```python
from build123d import *

# Parameters (mm, degrees)
SKETCH_1_R          = 3.073322802
EXTRUDE_1_DEPTH     = 10
SKETCH_2_R          = 3
EXTRUDE_2_DEPTH     = 5
CUT_EXTRUDE_1_DEPTH = 10


with BuildPart() as part:
    # 草图1 → 凸台-拉伸1 (new body)
    with BuildSketch(Plane(origin=(0, 0, 0), x_dir=(1, 0, 0), z_dir=(0, 1, 0))):
        with BuildLine():
            Line((0, 0), (30.73322802, 0))
            Line((30.73322802, 0), (18.141743603, 40.76055825))
            ThreePointArc((18.141743603, 40.76055825), (15.36661401, 42.513286949), (12.591484417, 40.76055825))
            Line((12.591484417, 40.76055825), (0, 0))
        make_face()
        with Locations(Location((15.36661401, 30, 0), (0, 0, 270))):
            Circle(SKETCH_1_R, mode=Mode.SUBTRACT)
    extrude(amount=EXTRUDE_1_DEPTH)

    # 草图2 → 凸台-拉伸2 (add)
    with BuildSketch(Plane.XZ):
        with Locations(Location((15.36661401, -39.439964147, 0), (0, 0, 90))):
            Circle(SKETCH_2_R)
    extrude(amount=EXTRUDE_2_DEPTH)

    # 草图3 → 切除-拉伸1 (cut)
    with BuildSketch(Plane(origin=(0, 10, 0), x_dir=(1, 0, 0), z_dir=(0, 1, 0))):
        with BuildLine():
            Line((13.327100422, 20.21204175), (13.327100422, 24.21204175))
            Line((13.327100422, 24.21204175), (17.327100422, 24.21204175))
            Line((17.327100422, 24.21204175), (17.327100422, 20.21204175))
            ThreePointArc((17.327100422, 20.21204175), (15.327100422, 0.414082779), (13.327100422, 20.21204175))
        make_face()
    extrude(amount=-CUT_EXTRUDE_1_DEPTH, mode=Mode.SUBTRACT)


solid = part.part
```
For this review, take the finished solid that the model builds, in its own axes (mm). A direction names the side the tool comes from. Coordinates: 2 decimals unless noted, no trailing zeros. Write each loop counter-clockwise with the first axis right and the second up, starting at its lowest first coordinate (ties: lowest second). Pieces come first, ordered by that corner, then holes. Notation, with made-up numbers: (89.25, 76) - (100.25, 76) arc R4 cw to (100.25, 82) - close; hole circle Ø10 at (35, 2). An arc over 180 degrees is marked (long way). Answer in a Markdown table with one row per item. Add a question column.
Q1. For probe 1 along Z at (x, y) = (16, 7.75); probe 2 along X at (y, z) = (0.75, -6); probe 3 along X at (y, z) = (2.5, -5.5), list the stretches that pass through material, from the lowest coordinate up.
Q2. For P1, Ø6, axis at y = 2.5, z = -38, coming from the -X side; P2, Ø1, axis at y = -2, z = -4.5, coming from the -X side; P3, Ø2, axis at y = 6, z = -22, coming from the +X side; P4, Ø1, axis at y = 0.5, z = -15, coming from the -X side, all flat-tipped, find the tip position at first contact; note any pin that passes through.
Q3. We need section D-D, the plane z = -37. State the section outline as (x, y) points, and give its area (3 significant figures).
Q4. Tool access review of faces 1 (the flat face through (15, -5, -39)), 2 (the cylindrical face through (15.235, -2.465, -42.437)), 3 (the flat face through (17.327, 5, -22)): name each direction out of +Z, -Z, +X, -X, +Y, -Y from which nothing blocks a thin tool from reaching the whole face with its end or side.
Q5. We need section C-C, the plane y = 7.5. State the section outline as (x, z) points, and give its area (3 significant figures).
Q6. We need section B-B, the plane z = -30. State the section outline as (x, y) points, and give its area (3 significant figures).
Q7. Draft analysis for pull direction X (two halves, no side actions). For faces 4 (the cylindrical face through (15.415, 4.93, -42.513)), 5 (the flat face through (15, 5, 0)), 6 (the flat face through (15, 5, -24.212)), 7 (the cylindrical face through (15.739, 5.07, -0.423)), state which applies: +X half, -X half, draft (parallel to the pull), parting line (faces both ways), or undercut.
Q8. We need section A-A, the plane x = 7. State the section outline as (y, z) points, and give its area (3 significant figures).
Answer list:
| question | item | result |
|---|---|---|
| 1 | probe 1 | z = -42.45 to -33.01, -26.99 to -24.21, -0.44 to 0 |
| 1 | probe 2 | x = 1.85 to 6.35, 24.3 to 28.88 |
| 1 | probe 3 | x = 1.7 to 6.62, 24.04 to 29.03 |
| 2 | P1 | stops at x = 10.81 |
| 2 | P2 | passes through |
| 2 | P3 | stops at x = 24.25 |
| 2 | P4 | stops at x = 4.48 |
| 3 | outline | (11.43, 0) - (13.62, 0) - (13.62, -5) - (17.11, -5) - (17.11, 0) - (19.3, 0) - (19.3, 10) - (11.43, 10) - close |
| 3 | area | 96.2 mm2 |
| 4 | face 1 | +Z, -Z, +X, -X, -Y |
| 4 | face 2 | -Y |
| 4 | face 3 | +Y, -Y |
| 5 | outline | (0, 0) - (12.59, -40.76) arc R3.07 ccw to (18.14, -40.76) - (30.73, 0) - close; hole circle Ø6.15 at (15.37, -30); hole (13.33, -24.21) - (17.33, -24.21) - (17.33, -20.21) arc R10 ccw (long way) to (13.33, -20.21) - close |
| 5 | area | 387 mm2 |
| 6 | outline | (9.27, 0) - (12.29, 0) - (12.29, 10) - (9.27, 10) - close; (18.44, 0) - (21.47, 0) - (21.47, 10) - (18.44, 10) - close |
| 6 | area | 60.5 mm2 |
| 7 | face 4 | parting line |
| 7 | face 5 | draft |
| 7 | face 6 | undercut |
| 7 | face 7 | undercut |
| 8 | outline | (0, -22.66) - (10, -22.66) - (10, -15.95) - (0, -15.95) - close; (0, -4.88) - (10, -4.88) - (10, 0) - (0, 0) - close |
| 8 | area | 116 mm2 |
